The model under review builds one solid part; all positions refer to its coordinate system, in mm. Face numbers are marked on the shaded views. A direction names the side the tool comes from. Round coordinates to 2 decimals unless told otherwise and drop trailing zeros. Loops run counter-clockwise (first coordinate to the right, second up) from the corner with the lowest first, then second, coordinate; pieces in that order, holes last. Notation, with made-up numbers: (60, 45) -> (79, 45) arc R32 ccw to (79, 73) -> close; hole circle Ø8 at (-10, 85.5). An arc over 180 degrees is marked (long way). Write each question's results on one line, items separated by ' | '. Start each with the question number.
Item 1: We need section D-D (x = -13.5). Give the boundary of the cut face in (y, z), and give its area (3 significant figures).
Item 2: We need section C-C (z = 15.5). Give the boundary of the cut face in (x, y).
Item 3: We need section B-B (y = 34.5). Give the boundary of the cut face in (x, z).
Item 4: Tool access review of the marked faces 4 and 5: name each direction out of +Z, -Z, +X, -X, +Y, -Y from which nothing blocks a thin tool from reaching the whole face with its end or side.
Item 5: We need section A-A (z = 0). Give the boundary of the cut face in (x, y).
Item 6: Clearance check with flat-ended pins moving along their axes: pin 1 Ø2 at (x, z) = (-5, -3.5) entering from +Y; pin 2 Ø2.5 at (y, z) = (23.38, 15.53) entering from +X; pin 3 Ø10 at (y, z) = (10, -11.5) entering from -X. State where each tip first meets the part, or that it passes through.
Item 7: For L1, parallel to X at y = 20, z = -15.5; L2, parallel to Y at x = -5, z = -12.5, list the stretches that pass through material, from the lowest coordinate up. Write a range as from..to.
Item 8: Mouldability with a two-part tool opening along Y and no side actions: class the marked faces 1, 2 and 3 as pulls with the +Y half, pulls with the -Y half, needs draft (parallel to the pull), parting line crosses it, or undercut.
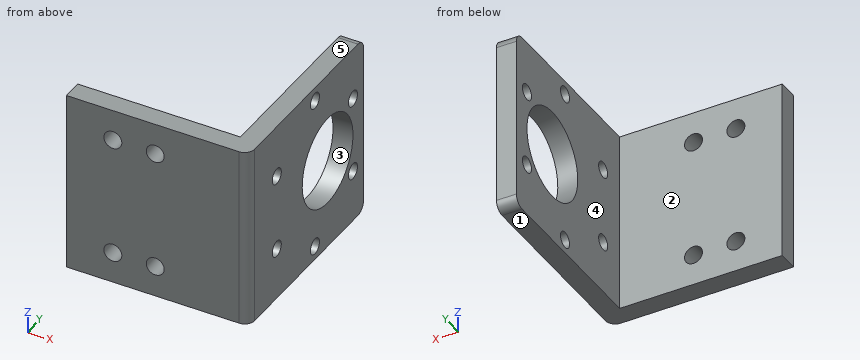
from build123d import *

# Parameters (mm, degrees)
SKETCH_1_W          = 36.6
SKETCH_1_H          = 36.6
EXTRUDE_1_DEPTH     = 40.6
SKETCH_2_W          = 32.6
SKETCH_2_H          = 36.6
CUT_EXTRUDE_1_DEPTH = 36.6
SKETCH_3_R          = 9
SKETCH_3_R_2        = 1.6
CUT_EXTRUDE_5_DEPTH = 36.6
FILLET_1_R          = 2
FILLET_2_R          = 2
SKETCH_7_R          = 1.8
CUT_EXTRUDE_6_DEPTH = 10


with BuildPart() as part:
    # 草图1 → 凸台-拉伸1 (new body)
    with BuildSketch(Plane(origin=(0, 0, 0), x_dir=(1, 0, 0), z_dir=(0, 1, 0))):
        Rectangle(SKETCH_1_W, SKETCH_1_H)
    extrude(amount=EXTRUDE_1_DEPTH)

    # 草图2 → 切除-拉伸1 (cut)
    with BuildSketch(Plane(origin=(0, 40.6, 0), x_dir=(1, 0, 0), z_dir=(0, 1, 0))):
        with Locations((-2, 0)):
            Rectangle(SKETCH_2_W, SKETCH_2_H)
    extrude(amount=-CUT_EXTRUDE_1_DEPTH, mode=Mode.SUBTRACT)

    # 草图3 → 切除-拉伸5 (cut)
    with BuildSketch(Plane(origin=(18.3, 0, 0), x_dir=(0, 0, -1), z_dir=(1, 0, 0))):
        with Locations((0, 27.863666333)):
            Circle(SKETCH_3_R)
        with Locations((-7.745235234, 36.863666333)):
            Circle(SKETCH_3_R_2)
        with Locations((7.745235234, 36.863666333)):
            Circle(SKETCH_3_R_2)
        with Locations((-15.529977583, 23.38009706)):
            Circle(SKETCH_3_R_2)
        with Locations((15.529977583, 23.38009706)):
            Circle(SKETCH_3_R_2)
        with Locations((7.745235234, 9.85104245)):
            Circle(SKETCH_3_R_2)
        with Locations((-7.718974262, 9.85104245)):
            Circle(SKETCH_3_R_2)
    extrude(amount=-CUT_EXTRUDE_5_DEPTH, mode=Mode.SUBTRACT)

    # 圆角1
    fillet_1_edges = [part.edges().sort_by_distance(p)[0] for p in [
        (18.3, 0, 0),
    ]]
    fillet(fillet_1_edges, radius=FILLET_1_R)

    # 圆角2
    fillet_2_edges = [part.edges().sort_by_distance(p)[0] for p in [
        (16.3, 40.6, 18.3),
        (16.3, 40.6, -18.3),
    ]]
    fillet(fillet_2_edges, radius=FILLET_2_R)

    # 草图7 → 切除-拉伸6 (cut)
    with BuildSketch(Plane(origin=(0, 0, 0), x_dir=(-1, 0, 0), z_dir=(0, -1, 0))):
        with Locations(Location((0.50738419, 12.025, 0), (0, 0, 90))):
            Circle(SKETCH_7_R)
        with Locations(Location((9.00738419, 12.025, 0), (0, 0, 90))):
            Circle(SKETCH_7_R)
        with Locations(Location((9.00738419, -12.025, 0), (0, 0, 270))):
            Circle(SKETCH_7_R)
        with Locations(Location((0.50738419, -12.025, 0), (0, 0, 270))):
            Circle(SKETCH_7_R)
    extrude(amount=-CUT_EXTRUDE_6_DEPTH, mode=Mode.SUBTRACT)


solid = part.part
Here are the results:
1) outline: (0, -18.3) -> (4, -18.3) -> (4, 18.3) -> (0, 18.3) -> close | area: 146 mm2
2) outline: (-18.3, 0) -> (16.3, 0) arc R2 ccw to (18.3, 2) -> (18.3, 21.78) -> (14.3, 21.78) -> (14.3, 4) -> (-18.3, 4) -> close; (14.3, 24.98) -> (18.3, 24.98) -> (18.3, 40.6) -> (14.3, 40.6) -> close
3) outline: (14.3, -18.3) -> (18.3, -18.3) -> (18.3, -6.08) -> (14.3, -6.08) -> close; (14.3, 6.08) -> (18.3, 6.08) -> (18.3, 18.3) -> (14.3, 18.3) -> close
4) face 4: +Z, -Z, -X, +Y | face 5: +Z, +X, -X, +Y, -Y
5) outline: (-18.3, 0) -> (16.3, 0) arc R2 ccw to (18.3, 2) -> (18.3, 18.86) -> (14.3, 18.86) -> (14.3, 4) -> (-18.3, 4) -> close; (14.3, 36.86) -> (18.3, 36.86) -> (18.3, 40.6) -> (14.3, 40.6) -> close
6) pin 1: stops at y = 4 | pin 2: passes through | pin 3: stops at x = 14.3
7) L1: x = 14.3..18.3 | L2: y = 0..4
8) face 1: needs draft | face 2: pulls with the +Y half | face 3: undercut
